Autodesk Inventor part; units mm, degrees
ref_plane "YZ Plane" through (0, 0, 0) normal (1, 0, 0) x (0, 1, 0)
ref_plane "XZ Plane" through (0, 0, 0) normal (0, 1, 0) x (-1, 0, 0)
ref_plane "XY Plane" through (0, 0, 0) normal (0, 0, 1) x (1, 0, 0)
sketch "Sketch3" plane through (0, 0, 0) normal (0, 1, 0) x (-1, 0, 0)
  line L0 (-14.9997, 0) -> (-19.9997, 0)
  line L1 (-19.9997, 0) -> (-19.9997, 15)
  line L2 (-19.9997, 15) -> (-14.9997, 15)
  line L3 (-14.9997, 15) -> (-14.9997, 0)
  line L4 (14.9998, 0) -> (19.9998, 0)
  line L5 (19.9998, 0) -> (19.9998, 15)
  line L6 (19.9998, 15) -> (14.9998, 15)
  line L7 (14.9998, 15) -> (14.9998, 0)
  point P0 (0, 0)
  dimension "d4" = 5
  dimension "d5" = 15
  dimension "d6" = 5
  dimension "d7" = 15
extrude "Extrusion1" add sketch "Sketch3" along normal blind 5
sketch "Sketch5" plane through (-19.9998, 0, 15) normal (0, 0, 1) x (1, 0, 0)
  line L0 (5, 0) -> (0, 0)
  line L1 (0, 0) -> (5, 0)
  line L2 (5, 0) -> (5, 2)
  line L3 (5, 2) -> (0, 2)
  line L4 (0, 2) -> (0, 0)
  line L5 (34.9995, 0) -> (39.9995, 0)
  line L6 (34.9995, 0) -> (39.9995, 0)
  line L7 (39.9995, 0) -> (39.9995, 2)
  line L8 (39.9995, 2) -> (34.9995, 2)
  line L9 (34.9995, 2) -> (34.9995, 0)
  point P0 (19.9998, 0)
  dimension "d10" = 5
  dimension "d11" = 2
  dimension "d12" = 5
  dimension "d13" = 2
extrude "Extrusion2" add sketch "Sketch5" along normal blind 3
sketch "Sketch6" plane through (-19.9998, 2, 15) normal (0, 1, 0) x (1, 0, 0)
  point P0 (19.9998, 15)
sketch "Sketch7" plane through (-19.9998, 2, 15) normal (0, 1, 0) x (1, 0, 0)
  circle A0 centre (2.5, -1.466) radius 1
  line L0 (0, 0) -> (0, -3)
  circle A1 centre (37.4995, -1.5) radius 1
  line L1 (34.9995, 0) -> (34.9995, -3)
  point P0 (19.9998, 15)
  point P1 (0, -1.5)
  point P2 (34.9995, -1.5)
  dimension "d16" = 2
  dimension "d17" = 2.5
  dimension "d18" = 2
  dimension "d19" = 2.5
extrude "Extrusion3" cut sketch "Sketch7" against normal blind 2
sketch "Sketch8" plane through (19.9997, 0, 0) normal (0, 0, -1) x (-1, 0, 0)
  line L0 (0, 2) -> (0, 5)
  line L1 (0, 2.5002) -> (40, 2.5002)
  line L2 (40, 2.5002) -> (40, -7.5998)
  line L3 (40, -7.5998) -> (0, -7.5998)
  line L4 (0, -7.5998) -> (0, 2.5002)
  point P0 (19.9997, 0)
  dimension "d22" = 40
  dimension "d23" = 10.1
extrude "Extrusion4" add sketch "Sketch8" along normal blind 2
sketch "Sketch9" plane through (19.9997, 0, 0) normal (0, 0, 1) x (1, 0, 0)
  line L0 (-40, -7.5998) -> (-40, 2.5002)
  line L1 (-40, -5.1) -> (-35, -5.1)
  line L2 (-35, -5.1) -> (-35, -10.1)
  line L3 (-35, -10.1) -> (-40, -10.1)
  line L4 (-40, -10.1) -> (-40, -5.1)
  line L5 (0, 0) -> (0, -7.5998)
  line L6 (0, -5.1) -> (-5, -5.1)
  line L7 (-5, -5.1) -> (-5, -10.1)
  line L8 (-5, -10.1) -> (0, -10.1)
  line L9 (0, -10.1) -> (0, -5.1)
  point P0 (-19.9997, 0)
  dimension "d26" = 5
  dimension "d27" = 5
  dimension "d28" = 5
  dimension "d29" = 5
extrude "Extrusion5" add sketch "Sketch9" along normal blind 15
sketch "Sketch10" plane through (19.9997, 0, 15) normal (0, 0, 1) x (1, 0, 0)
  line L0 (-35, -5.1) -> (-40, -5.1)
  line L1 (-40, -5.1) -> (-40, -7.1)
  line L2 (-40, -7.1) -> (-35, -7.1)
  line L3 (-35, -7.1) -> (-35, -5.1)
  line L4 (-5, -5.1) -> (-5, -10.1)
  line L5 (-5, -5.1) -> (0, -5.1)
  line L6 (0, -5.1) -> (0, -7.1)
  line L7 (0, -7.1) -> (-5, -7.1)
  line L8 (-5, -7.1) -> (-5, -5.1)
  point P0 (-19.9997, 0)
  dimension "d32" = 5
  dimension "d33" = 2
  dimension "d34" = 5
  dimension "d35" = 2
extrude "Extrusion6" add sketch "Sketch10" along normal blind 3
sketch "Sketch11" plane through (-20.0003, -7.1, 15) normal (0, -1, 0) x (1, 0, 0)
  circle A0 centre (2.4996, 1.4564) radius 1
  line L0 (0, 0) -> (0, 3)
  circle A1 centre (37.5, 1.4063) radius 1
  line L1 (40, 0) -> (40, 3)
  point P0 (20.0003, -15)
  point P1 (0, 1.5)
  point P2 (40, 1.5)
  dimension "d38" = 2
  dimension "d39" = 2.5
  dimension "d40" = 2
  dimension "d41" = 2.5
extrude "Extrusion7" cut sketch "Sketch11" against normal blind 2
sketch "Sketch13" plane through (19.9997, 5, 15) normal (1, 0, 0) x (0, 0, -1)
  circle A0 centre (20.3727, -7.5498) radius 5
  point P0 (15, -5)
  dimension "d44" = 10
extrude "Extrusion8" add sketch "Sketch13" against normal blind 2
sketch "Sketch14" plane through (17.9997, 5, 15) normal (-1, 0, 0) x (0, 0, 1)
  arc A0 (-17, -3.8586) -> (-17, -11.241) centre (-20.3727, -7.5498) ccw
  point P0 (-15, -5)
sketch "Sketch15" plane through (-20.0003, -7.5998, -2) normal (-1, 0, 0) x (0, 0, 1)
  point P0 (2, 7.5998)
sketch "Sketch16" plane through (-20.0003, -7.5998, -2) normal (-1, 0, 0) x (0, 0, 1)
  circle A0 centre (-3.3725, 5.0498) radius 5
  point P0 (2, 7.5998)
  dimension "d47" = 10
extrude "Extrusion9" add sketch "Sketch16" against normal blind 2
sketch "Sketch18" plane through (-20.0003, 2.5002, -2) normal (-1, 0, 0) x (0, 0, 1)
  arc A0 (0, -1.3588) -> (0, -8.7412) centre (-3.3727, -5.05) ccw
  circle A1 centre (-3.3727, -5.05) radius 3.5
  point P0 (2, -2.5002)
  dimension "d50" = 7
extrude "Extrusion10" cut sketch "Sketch18" against normal blind 40
properties part number "mount"
Work out the finished part from the listing and answer in its coordinate system (mm). A direction names the side the tool comes from. Give positions to 0.01 mm unless a question says otherwise; leave off trailing zeros. Order: outer loops, then holes, each group sorted by start corner. A loop starts at its lowest first (then second) coordinate and runs counter-clockwise, first axis right, second up. Notation, with made-up numbers: M 50.25,64.25 L 95.25,64.25 A14 cw 95.25,80.25 Z; hole C 25,-13.5 d1. An arc over 180 degrees is marked long. Return JSON: item names as keys, results as strings.
Q1. Find section C-C, the plane y = -0.75. Write down the section's boundary in (x, z), and give its area (3 significant figures).
Answer below:
{"outline": "M -20,-10.04 L -18,-10.04 L -18,-8.37 L -20,-8.37 Z; M -20,-2.37 L -18,-2.37 L -18,-2 L 18,-2 L 18,-2.37 L 20,-2.37 L 20,0 L -20,0 Z; M 18,-10.04 L 20,-10.04 L 20,-8.37 L 18,-8.37 Z", "area": "88.1 mm^2"}
Q2. Each of these flat-tipped pins is pushed along its axis until it touches: pin 1 (1.5 mm diameter, centred on x = 17.5, y = -8, fed in from +Z); pin 2 (0.6 mm diameter, centred on x = 8, z = -1, fed in from -Y); pin 3 (2 mm diameter, centred on x = 11.5, z = -1, fed in from +Y); pin 4 (6 mm diameter, centred on y = -4, z = 1.5, fed in from -X). Where does it stop, or does it pass through?
Answer below:
{"pin 1": "stops at z = 15", "pin 2": "stops at y = -7.6", "pin 3": "stops at y = 2.5", "pin 4": "stops at x = -20"}
Q3. Find section A-A, the plane z = 1. Write down the section's boundary in (x, y).
Answer below:
{"outline": "M -20,-10.1 L -15,-10.1 L -15,-5.1 L -20,-5.1 Z; M -20,0 L -15,0 L -15,5 L -20,5 Z; M 15,-10.1 L 20,-10.1 L 20,-5.1 L 15,-5.1 Z; M 15,0 L 20,0 L 20,5 L 15,5 Z"}
Q4. Which of the six approach directions +Z, -Z, +X, -X, +Y, -Y give full straight-line access (tool end or side, diameter ignored) to faces 5 (the face through (0, -2, 0)), 6 (the face through (-17, 0, 9)), 7 (the face through (16, 2, 16)), 8 (the face through (0, 2.5, -1))?
Answer below:
{"face 5": "+Z", "face 6": "+Z, +X, -X", "face 7": "+Z, +X, -X, +Y", "face 8": "-Z, +X, -X, +Y"}
Q5. Find section D-D, the plane x = -4. Write down the section's boundary in (y, z).
Answer below:
{"outline": "M -7.6,-2 L -3.49,-2 A3.5 cw -1.61,-2 L 2.5,-2 L 2.5,0 L -7.6,0 Z"}
Q6. Find the intervals of material crossed by line 1 along X through (y, z) = (0.8, 16.5); line 2 along X through (y, z) = (-5.75, 12.75); line 3 along X through (y, z) = (1.5, -8), in increasing order. Write a range as [from, to].
Answer below:
{"line 1": "x = [-20, -18.5], [-16.5, -15], [15, 16.5], [18.5, 20]", "line 2": "x = [-20, -15], [15, 20]", "line 3": "x = [-20, -18], [18, 20]"}
Q7. The mould has two halves that part along Z. Classify faces 1 (the face through (-17.038, 1.014, 17.353)), 2 (the face through (-18, -9, 15)), 3 (the face through (-17, 4, 0)), 4 (the face through (-17, -10.1, 7)): pulls with the +Z half, pulls with the -Z half, needs draft (parallel to the pull), parting line crosses it, or undercut.
Answer below:
{"face 1": "undercut", "face 2": "pulls with the +Z half", "face 3": "pulls with the -Z half", "face 4": "needs draft"}
Q8. Find section B-B, the plane y = -8.25. Write down the section's boundary in (x, z), and give its area (3 significant figures).
Answer below:
{"outline": "M -20,0 L -15,0 L -15,15 L -20,15 Z; M 15,0 L 20,0 L 20,15 L 15,15 Z", "area": "150 mm^2"}
